Check sheet for the modelled part. Datum: model origin and axes. Units: mm. A direction names the side the tool comes from. Give positions to 0.01 mm unless a question says otherwise; leave off trailing zeros. Order: outer loops, then holes, each group sorted by start corner. A loop starts at its lowest first (then second) coordinate and runs counter-clockwise, first axis right, second up. Notation, with made-up numbers: (21.25, 34) -> (58.25, 34) arc R17 ccw to (58.25, 43) -> close; hole circle Ø2 at (-6.75, 2). An arc over 180 degrees is marked (long way). One line per question, with ' | ' between items.
```python
from build123d import *
from build123d import SkipClean  # not in build123d's __all__

# Parameters (mm, degrees)
F0_R     = 10
F1_DEPTH = 2.5
F3_DEPTH = 3
F4_DEPTH = 25


# Not quite as in the source:
# - a feature names something its author has since deleted; it is built from what else it names


with BuildPart() as f1:
    # F0 (on Top) → F1 (new body, symmetric)
    with BuildSketch(Plane.XY):
        with BuildLine():
            Line((-3, 50.3508893593), (-3, -50.3508893593))
            ThreePointArc((-3, -50.3508893593), (1.5102254254, -75.9119796764), (0, -50))
            Line((0, -50), (0, 50))
            ThreePointArc((0, 50), (1.5102254254, 75.9119796764), (-3, 50.3508893593))
        make_face()
        with Locations((0, -63)):
            Circle(F0_R, mode=Mode.SUBTRACT)
        with Locations((0, 63)):
            Circle(F0_R, mode=Mode.SUBTRACT)
    extrude(amount=F1_DEPTH, both=True)

    # F2 (on face) → F3 (join, through all)
    with BuildSketch(Plane.YZ):
        with BuildLine():
            ThreePointArc((-3.4641016151, 2.5), (-1.0352761804, 8.3637033052), (4, 4.5))
            ThreePointArc((4, 4.5), (3.8637033052, 3.4647238196), (3.4641016151, 2.5))
            Line((3.4641016151, 2.5), (13.0766968306, 2.5))
            ThreePointArc((13.0766968306, 2.5), (9.108069864, 3.7337187027), (6.5383484153, 7))
            ThreePointArc((6.5383484153, 7), (0, 11.5), (-6.5383484153, 7))
            ThreePointArc((-6.5383484153, 7), (-9.108069864, 3.7337187027), (-13.0766968306, 2.5))
            Line((-13.0766968306, 2.5), (-3.4641016151, 2.5))
        make_face()
        with BuildLine():
            ThreePointArc((3.4641016151, 2.5), (0, 0.5), (-3.4641016151, 2.5))
            Line((-3.4641016151, 2.5), (-13.0766968306, 2.5))
            Line((-13.0766968306, 2.5), (-13.0766968306, -2.5))
            Line((-13.0766968306, -2.5), (13.0766968306, -2.5))
            Line((13.0766968306, -2.5), (13.0766968306, 2.5))
            Line((13.0766968306, 2.5), (3.4641016151, 2.5))
        make_face()
    extrude(amount=-F3_DEPTH)

    # F2 (on face) → F4 (cut)
    with BuildSketch(Plane.YZ):
        with BuildLine():
            Line((3.4641016151, 2.5), (-3.4641016151, 2.5))
            ThreePointArc((-3.4641016151, 2.5), (0, 0.5), (3.4641016151, 2.5))
        make_face()
    with SkipClean():  # cleaning this boolean's faces spoils the solid; the shape is the same uncleaned
        extrude(amount=-F4_DEPTH, mode=Mode.SUBTRACT)


solid = f1.part
```
Q1. Access from +Z, -Z, +X, -X, +Y, -Y to the whole of each face (thin tool, end or side, straight path). Record for faces 1 (the face through (-3, 0, 0)), 2 (the face through (0, 0, 0)), 3 (the face through (-1, -49, 2.5)), 4 (the face through (-1, 0, -2.5)).
Result sheet:
face 1: +Z, -Z, -X | face 2: +Z, -Z, +X | face 3: +Z, +X, -X, -Y | face 4: -Z, +X, -X, +Y, -Y
Q2. Section check B-B (y = -63). Enter the section's corners in (x, z).
Result sheet:
outline: (-13, -2.5) -> (-10, -2.5) -> (-10, 2.5) -> (-13, 2.5) -> close; (10, -2.5) -> (13, -2.5) -> (13, 2.5) -> (10, 2.5) -> close
Q3. Thickness scan on line 1 (Y direction, x = 2, z = -1.5); line 2 (X direction, y = -25.5, z = 0); line 3 (Z direction, x = 10, y = 65). Record the ranges inside material, lowest first.
Result sheet:
line 1: y = -75.85 to -72.8, -53.2 to -50.15, 50.15 to 53.2, 72.8 to 75.85 | line 2: x = -3 to 0 | line 3: z = -2.5 to 2.5
Q4. Section check A-A (y = 0). Enter the section's corners in (x, z), and give its area (3 significant figures).
Result sheet:
outline: (-3, -2.5) -> (0, -2.5) -> (0, 0.5) -> (-3, 0.5) -> close; (-3, 8.5) -> (0, 8.5) -> (0, 11.5) -> (-3, 11.5) -> close | area: 18.0 mm2
Q5. Mould release check, pull along Y, two halves, no side actions. Record for faces 5 (the face through (-2.17, 53.24, -0.04)), 6 (the face through (-1, 49, 2.5)), 7 (the face through (0.962, -75.964, 0.035)): pulls with the +Y half, pulls with the -Y half, needs draft (parallel to the pull), parting line crosses it, or undercut.
Result sheet:
face 5: undercut | face 6: needs draft | face 7: undercut
Q6. Section check C-C (z = 10.25). Enter the section's corners in (x, y).
Result sheet:
outline: (-3, -3.99) -> (0, -3.99) -> (0, 3.99) -> (-3, 3.99) -> close
Q7. Depth check by flat-ended pin: pin 1 Ø7 at (y, z) = (19, 1) entering from -X; pin 2 Ø6 at (x, z) = (-3.5, 4) entering from +Y; pin 3 Ø6 at (x, z) = (-8, 4) entering from +Y. Enter the tip coordinate at first touch or a pass-through.
Result sheet:
pin 1: stops at x = -3 | pin 2: stops at y = 75.97 | pin 3: stops at y = 74.82
Q8. Section check D-D (y = -29). Enter the section's corners in (x, z), and give its area (3 significant figures).
Result sheet:
outline: (-3, -2.5) -> (0, -2.5) -> (0, 2.5) -> (-3, 2.5) -> close | area: 15.0 mm2
